Read the model definition and answer for the solid it produces. Units are mm, in the model's axes. A direction names the side the tool comes from. Give positions to 0.01 mm unless a question says otherwise; leave off trailing zeros. Loops run counter-clockwise (first coordinate to the right, second up) from the corner with the lowest first, then second, coordinate; pieces in that order, holes last. Notation, with made-up numbers: (-6.5, 51) -> (49.5, 51) arc R26 cw to (49.5, 83) -> close; hole circle Ø3 at (-38.5, -39.75). An arc over 180 degrees is marked (long way). Write each question's results on one line, items separated by ' | '. Start each with the question number.
Item 1: Which of the six approach directions +Z, -Z, +X, -X, +Y, -Y give full straight-line access (tool end or side, diameter ignored) to faces 1 (the flat face through (32.353, 15, 63)), 2 (the flat face through (2, 17, 40.712)), 3 (the flat face through (37, 6.466, 21))?
Item 2: Determine the mould class of faces 4 (the flat face through (2, 15, -4.288)), 5 (the flat face through (-7, 30, 44)), 6 (the flat face through (31.353, 28, 21)) for opening direction Z: +Z half, -Z half, draft (parallel to the pull), parting line (faces both ways), or undercut.
Item 3: Section B-B on z = 67 is taken. Write down the section's boundary in (x, y).
Item 4: Find the intervals of material crossed by line 1 (Z direction, x = -26, y = 16.75); line 2 (Z direction, x = 28, y = 26.5); line 3 (X direction, y = 19.5, z = 55), in increasing order.
Item 5: Section D-D on x = 35 is taken. Write down the section's boundary in (y, z).
Item 6: Section A-A on y = 13 is taken. Write down the section's boundary in (x, z).
Item 7: Section C-C on x = 25 is taken. Write down the section's boundary in (y, z), and give its area (3 significant figures).
Item 8: Each of these flat-tipped pins is pushed along its axis until it touches: P1, Ø1, axis at x = 3.5, y = 22.5, coming from the +Z side; P2, Ø5, axis at x = 8, z = 66, coming from the +Y side. Where does it stop, or does it pass through?
```python
from build123d import *

# Parameters (mm, degrees)
SKETCH2_W          = 80
SKETCH2_H          = 100
SKETCH2_R          = 10
CAMERA_LENSE_DEPTH = 5
SKETCH3_W          = 80
SKETCH3_H          = 100
SKETCH3_W_2        = 58
SKETCH3_H_2        = 40
SKETCH3_W_3        = 60
SKETCH3_H_3        = 35
CAMERA_DEPTH       = 25
HOLLOW_START       = -2
SKETCH4_W          = 78
SKETCH4_H          = 27.979664862
HOLLOW_TOP_DEPTH   = 8
SKETCH10_W         = 80
SKETCH10_H         = 10
CUT_EXTRUDE4_DEPTH = 101.201733938
SKETCH11_W         = 30
SKETCH11_H         = 20
CUT_EXTRUDE5_DEPTH = 122.023203799
SKETCH12_W         = 20
SKETCH12_H         = 35
CUT_EXTRUDE6_DEPTH = 99.819975127
SKETCH13_W         = 55
SKETCH13_H         = 25
CUT_EXTRUDE7_DEPTH = 10


with BuildPart() as part:
    # Sketch2 → camera lense (new body)
    with BuildSketch(Plane(origin=(0, 0, 0), x_dir=(1, 0, 0), z_dir=(0, 1, 0))):
        with Locations((2.352941176, -35.712402007)):
            Rectangle(SKETCH2_W, SKETCH2_H)
        with Locations(Location((16.352941176, -25.712402007, 0), (0, 0, 270))):
            Circle(SKETCH2_R, mode=Mode.SUBTRACT)
    extrude(amount=CAMERA_LENSE_DEPTH)

    # Sketch3 → camera (add)
    with BuildSketch(Plane(origin=(0, 5, 0), x_dir=(1, 0, 0), z_dir=(0, 1, 0))):
        with Locations((2.352941176, -35.712402007)):
            Rectangle(SKETCH3_W, SKETCH3_H)
        with Locations((2.352941176, -20.712402007)):
            Rectangle(SKETCH3_W_2, SKETCH3_H_2, mode=Mode.SUBTRACT)
        with Locations((2.352941176, -63.212402007)):
            Rectangle(SKETCH3_W_3, SKETCH3_H_3, mode=Mode.SUBTRACT)
    extrude(amount=CAMERA_DEPTH)

    # Sketch4 → hollow top (cut)
    with BuildSketch(Plane(origin=(0, 0, -14.287597993), x_dir=(-1, 0, 0), z_dir=(0, 0, -1)).offset(HOLLOW_START)):
        with Locations((-2.352941176, 14.989832431)):
            Rectangle(SKETCH4_W, SKETCH4_H)
    extrude(amount=-HOLLOW_TOP_DEPTH, mode=Mode.SUBTRACT)

    # Sketch10 → Cut-Extrude4 (cut, through all)
    with BuildSketch(Plane(origin=(0, 30, 0), x_dir=(1, 0, 0), z_dir=(0, 1, 0))):
        with Locations((2.352941176, 9.287597993)):
            Rectangle(SKETCH10_W, SKETCH10_H)
    extrude(amount=-CUT_EXTRUDE4_DEPTH, mode=Mode.SUBTRACT)

    # Sketch11 → Cut-Extrude5 (cut, through all)
    with BuildSketch(Plane(origin=(42.352941176, 0, 0), x_dir=(0, 0, -1), z_dir=(1, 0, 0))):
        with Locations((-20.712402007, 16.465766073)):
            Rectangle(SKETCH11_W, SKETCH11_H)
    extrude(amount=-CUT_EXTRUDE5_DEPTH, mode=Mode.SUBTRACT)

    # Sketch12 → Cut-Extrude6 (cut, through all)
    with BuildSketch(Plane(origin=(0, 5, 0), x_dir=(1, 0, 0), z_dir=(0, 1, 0))):
        with Locations((22.352941176, -63.212402007)):
            Rectangle(SKETCH12_W, SKETCH12_H)
    extrude(amount=-CUT_EXTRUDE6_DEPTH, mode=Mode.SUBTRACT)

    # Sketch13 → Cut-Extrude7 (cut)
    with BuildSketch(Plane.XY.offset(85.712402007)):
        with Locations((2.352941176, 17.5)):
            Rectangle(SKETCH13_W, SKETCH13_H)
    extrude(amount=-CUT_EXTRUDE7_DEPTH, mode=Mode.SUBTRACT)


solid = part.part
```
Findings:
1) face 1: +Y, -Y | face 2: +Y | face 3: +X, -X
2) face 4: -Z half | face 5: draft | face 6: undercut
3) outline: (-37.65, 0) -> (12.35, 0) -> (12.35, 5) -> (-27.65, 5) -> (-27.65, 30) -> (-37.65, 30) -> close; (32.35, 0) -> (42.35, 0) -> (42.35, 30) -> (32.35, 30) -> close
4) line 1: -4.29 to 0.71, 40.71 to 45.71, 80.71 to 85.71 | line 2: -4.29 to 0.71, 40.71 to 45.71 | line 3: -37.65 to -27.65, 32.35 to 42.35
5) outline: (0, -4.29) -> (30, -4.29) -> (30, 85.71) -> (0, 85.71) -> close; hole (6.47, 5.71) -> (26.47, 5.71) -> (26.47, 35.71) -> (6.47, 35.71) -> close
6) outline: (-37.65, -4.29) -> (42.35, -4.29) -> (42.35, 5.71) -> (31.35, 5.71) -> (31.35, 0.71) -> (-26.65, 0.71) -> (-26.65, 5.71) -> (-37.65, 5.71) -> close; (-37.65, 35.71) -> (-26.65, 35.71) -> (-26.65, 40.71) -> (31.35, 40.71) -> (31.35, 35.71) -> (42.35, 35.71) -> (42.35, 85.71) -> (29.85, 85.71) -> (29.85, 80.71) -> (32.35, 80.71) -> (32.35, 45.71) -> (-27.65, 45.71) -> (-27.65, 80.71) -> (-25.15, 80.71) -> (-25.15, 85.71) -> (-37.65, 85.71) -> close
7) outline: (0, -4.29) -> (30, -4.29) -> (30, 0.71) -> (5, 0.71) -> (5, 20.69) -> (0, 20.69) -> close; (0, 30.74) -> (5, 30.74) -> (5, 40.71) -> (30, 40.71) -> (30, 45.71) -> (0, 45.71) -> close; (0, 80.71) -> (5, 80.71) -> (5, 85.71) -> (0, 85.71) -> close | area: 475 mm2
8) P1: z = 45.71 | P2: y = 5
